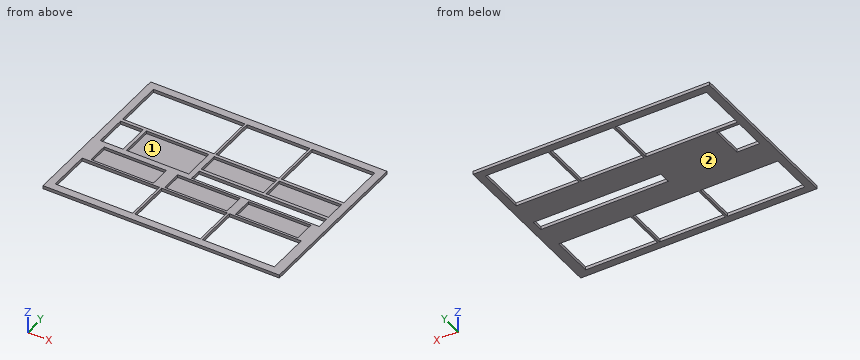
from build123d import *

# Parameters (mm, degrees)
SKETCH_1_W          = 220
SKETCH_1_H          = 160
EXTRUDE_1_DEPTH     = 3
SKETCH_2_W          = 85
SKETCH_2_H          = 46
SKETCH_2_W_2        = 58.5
CUT_EXTRUDE_1_DEPTH = 137.047785723
CUT_EXTRUDE_2_REACH = 138.048
SKETCH_3_W          = 21.2
SKETCH_3_H          = 30
SKETCH_4_W          = 58
SKETCH_4_H          = 30
SKETCH_4_H_2        = 19.5
CUT_EXTRUDE_3_DEPTH = 2.6
SKETCH_6_W          = 118.75
SKETCH_6_H          = 11
CUT_EXTRUDE_4_DEPTH = 137.047785723
CUT_EXTRUDE_5_REACH = 138.048
SKETCH_7_W          = 72
SKETCH_7_H          = 40
SKETCH_7_W_2        = 61
SKETCH_7_W_3        = 67
SKETCH_8_W          = 58
SKETCH_8_H          = 19.5
CUT_EXTRUDE_6_DEPTH = 2.6


with BuildPart() as part:
    # 草图1 → 凸台-拉伸1 (new body)
    with BuildSketch(Plane.XY):
        Rectangle(SKETCH_1_W, SKETCH_1_H)
    extrude(amount=EXTRUDE_1_DEPTH)

    # 草图2 → 切除-拉伸1 (cut, through all)
    with BuildSketch(Plane.XY.offset(3)):
        with Locations((-60.5, 50)):
            Rectangle(SKETCH_2_W, SKETCH_2_H)
        with Locations((13.25, 50)):
            Rectangle(SKETCH_2_W_2, SKETCH_2_H)
        with Locations((73.75, 50)):
            Rectangle(SKETCH_2_W_2, SKETCH_2_H)
    extrude(amount=-CUT_EXTRUDE_1_DEPTH, mode=Mode.SUBTRACT)

    # 草图3 → 切除-拉伸2 (cut, up to next)
    with BuildSketch(Plane.XY.offset(3), mode=Mode.PRIVATE) as cut_extrude_2_sk1:
        with Locations((-92.4, 9)):
            Rectangle(SKETCH_3_W, SKETCH_3_H)
    cut_extrude_2_tool1 = extrude(cut_extrude_2_sk1.sketch, amount=-CUT_EXTRUDE_2_REACH, mode=Mode.PRIVATE) & part.part
    add(cut_extrude_2_tool1.solids().sort_by_distance((-92.4, 9, 3))[0], mode=Mode.SUBTRACT)

    # 草图4 → 切除-拉伸3 (cut)
    with BuildSketch(Plane.XY.offset(3)):
        with Locations((-49.8, 9)):
            Rectangle(SKETCH_4_W, SKETCH_4_H)
        with Locations((13.25, 14.25)):
            Rectangle(SKETCH_4_W, SKETCH_4_H_2)
        with Locations((73.75, 14.25)):
            Rectangle(SKETCH_4_W, SKETCH_4_H_2)
    extrude(amount=-CUT_EXTRUDE_3_DEPTH, mode=Mode.SUBTRACT)

    # 草图6 → 切除-拉伸4 (cut, through all)
    with BuildSketch(Plane.XY.offset(3)):
        with Locations((43.625, -4)):
            Rectangle(SKETCH_6_W, SKETCH_6_H)
    extrude(amount=-CUT_EXTRUDE_4_DEPTH, mode=Mode.SUBTRACT)

    # 草图7 → 切除-拉伸5 (cut, up to next)
    with BuildSketch(Plane.XY.offset(3), mode=Mode.PRIVATE) as cut_extrude_5_sk1:
        with Locations((-67, -53)):
            Rectangle(SKETCH_7_W, SKETCH_7_H)
    cut_extrude_5_tool1 = extrude(cut_extrude_5_sk1.sketch, amount=-CUT_EXTRUDE_5_REACH, mode=Mode.PRIVATE) & part.part
    # 草图7 → 切除-拉伸5 (cut, up to next)
    with BuildSketch(Plane.XY.offset(3), mode=Mode.PRIVATE) as cut_extrude_5_sk2:
        with Locations((1.5, -53)):
            Rectangle(SKETCH_7_W_2, SKETCH_7_H)
    cut_extrude_5_tool2 = extrude(cut_extrude_5_sk2.sketch, amount=-CUT_EXTRUDE_5_REACH, mode=Mode.PRIVATE) & part.part
    # 草图7 → 切除-拉伸5 (cut, up to next)
    with BuildSketch(Plane.XY.offset(3), mode=Mode.PRIVATE) as cut_extrude_5_sk3:
        with Locations((67.5, -53)):
            Rectangle(SKETCH_7_W_3, SKETCH_7_H)
    cut_extrude_5_tool3 = extrude(cut_extrude_5_sk3.sketch, amount=-CUT_EXTRUDE_5_REACH, mode=Mode.PRIVATE) & part.part
    add(cut_extrude_5_tool1.solids().sort_by_distance((-67, -53, 3))[0], mode=Mode.SUBTRACT)
    add(cut_extrude_5_tool2.solids().sort_by_distance((1.5, -53, 3))[0], mode=Mode.SUBTRACT)
    add(cut_extrude_5_tool3.solids().sort_by_distance((67.5, -53, 3))[0], mode=Mode.SUBTRACT)

    # 草图8 → 切除-拉伸6 (cut)
    with BuildSketch(Plane.XY.offset(3)):
        with Locations((-67, -21.25)):
            Rectangle(SKETCH_8_W, SKETCH_8_H)
        with Locations((1.5, -21.25)):
            Rectangle(SKETCH_8_W, SKETCH_8_H)
        with Locations((67.5, -21.25)):
            Rectangle(SKETCH_8_W, SKETCH_8_H)
    extrude(amount=-CUT_EXTRUDE_6_DEPTH, mode=Mode.SUBTRACT)


solid = part.part
Design review of the part built by this model. Coordinates are the model's own, in mm. Face numbers are marked on the shaded views. Coordinates: 2 decimals unless noted, no trailing zeros. Loops run counter-clockwise (first coordinate to the right, second up) from the corner with the lowest first, then second, coordinate; pieces in that order, holes last.
Item 1: Wall thickness on L1, parallel to Y at x = -92.5, z = 2.6; L2, parallel to X at y = -36, z = 2.2; L3, parallel to Y at x = 43, z = 2.9: over which ranges is each line inside the solid? List them lowest first.
Completed:
L1: y = -80 to -73, -33 to -31, -11.5 to -6, 24 to 27, 73 to 80
L2: x = -110 to -103, -31 to -29, 32 to 34, 101 to 110
L3: y = -80 to -73, -33 to -31, -11.5 to -9.5, 1.5 to 80
Item 2: Add section C-C (y = -64.5). Write out the cut boundary in (x, z), and give its area (3 significant figures).
Completed:
outline: (-110, 0) - (-103, 0) - (-103, 3) - (-110, 3) - close; (-31, 0) - (-29, 0) - (-29, 3) - (-31, 3) - close; (32, 0) - (34, 0) - (34, 3) - (32, 3) - close; (101, 0) - (110, 0) - (110, 3) - (101, 3) - close
area: 60.0 mm2
Item 3: Add section B-B (x = -76.5). Write out the cut boundary in (y, z).
Completed:
outline: (-80, 0) - (-73, 0) - (-73, 3) - (-80, 3) - close; (-33, 0) - (27, 0) - (27, 3) - (24, 3) - (24, 0.4) - (-6, 0.4) - (-6, 3) - (-11.5, 3) - (-11.5, 0.4) - (-31, 0.4) - (-31, 3) - (-33, 3) - close; (73, 0) - (80, 0) - (80, 3) - (73, 3) - close
Item 4: Add section A-A (y = 14). Write out the cut boundary in (x, z), and give its area (3 significant figures).
Completed:
outline: (-110, 0) - (-103, 0) - (-103, 3) - (-110, 3) - close; (-81.8, 0) - (110, 0) - (110, 3) - (102.75, 3) - (102.75, 0.4) - (44.75, 0.4) - (44.75, 3) - (42.25, 3) - (42.25, 0.4) - (-15.75, 0.4) - (-15.75, 3) - (-20.8, 3) - (-20.8, 0.4) - (-78.8, 0.4) - (-78.8, 3) - (-81.8, 3) - close
area: 144 mm2
Item 5: Add section D-D (x = 17.5). Write out the cut boundary in (y, z).
Completed:
outline: (-80, 0) - (-73, 0) - (-73, 3) - (-80, 3) - close; (-33, 0) - (-9.5, 0) - (-9.5, 3) - (-11.5, 3) - (-11.5, 0.4) - (-31, 0.4) - (-31, 3) - (-33, 3) - close; (1.5, 0) - (27, 0) - (27, 3) - (24, 3) - (24, 0.4) - (4.5, 0.4) - (4.5, 3) - (1.5, 3) - close; (73, 0) - (80, 0) - (80, 3) - (73, 3) - close
Item 6: Draft analysis for pull direction X (two halves, no side actions). For the marked faces 1 and 2, state which applies: pulls with the +X half, pulls with the -X half, needs draft (parallel to the pull), parting line crosses it, or undercut.
Completed:
face 1: undercut
face 2: needs draft
Item 7: Clearance check with a flat-ended pin moving along its axis: pin 1 (10 mm diameter, centred on x = -62.5, y = -22, fed in from +Z). State where the tip first meets the part, or that it passes through.
Completed:
pin 1: stops at z = 0.4
